from build123d import *

# Parameters (mm, degrees)
SKETCH1_W            = 25.4
SKETCH1_H            = 25.4
BOSS_EXTRUDE1_DEPTH  = 340.36
SKETCH2_W            = 22.225
SKETCH2_H            = 22.225
CUT_EXTRUDE1_DEPTH   = 681.72
SKETCH3_R            = 2.38125
CUT_EXTRUDE2_DEPTH   = 26.4
M6_CLEARANCE_HOLE1_D = 6.6


with BuildPart() as part:
    # Sketch1 → Boss-Extrude1 (new body, symmetric)
    with BuildSketch(Plane.XY):
        Rectangle(SKETCH1_W, SKETCH1_H)
    extrude(amount=BOSS_EXTRUDE1_DEPTH, both=True)

    # Sketch2 → Cut-Extrude1 (cut, through all)
    with BuildSketch(Plane.XY.offset(340.36)):
        Rectangle(SKETCH2_W, SKETCH2_H)
    extrude(amount=-CUT_EXTRUDE1_DEPTH, mode=Mode.SUBTRACT)

    # Sketch3 → Cut-Extrude2 (cut, through all)
    with BuildSketch(Plane(origin=(0, 12.7, 0), x_dir=(1, 0, 0), z_dir=(0, 1, 0))):
        with Locations((0, -215.9)):
            Circle(SKETCH3_R)
        with Locations((0, -203.2)):
            Circle(SKETCH3_R)
        with Locations((0, -190.5)):
            Circle(SKETCH3_R)
        with Locations((0, -177.8)):
            Circle(SKETCH3_R)
        with Locations((0, -165.1)):
            Circle(SKETCH3_R)
        with Locations((0, -152.4)):
            Circle(SKETCH3_R)
        with Locations((0, -139.7)):
            Circle(SKETCH3_R)
        with Locations((0, 139.7)):
            Circle(SKETCH3_R)
        with Locations((0, 152.4)):
            Circle(SKETCH3_R)
        with Locations((0, 165.1)):
            Circle(SKETCH3_R)
        with Locations((0, 177.8)):
            Circle(SKETCH3_R)
        with Locations((0, 190.5)):
            Circle(SKETCH3_R)
        with Locations((0, 215.9)):
            Circle(SKETCH3_R)
        with Locations((0, 203.2)):
            Circle(SKETCH3_R)
    extrude(amount=-CUT_EXTRUDE2_DEPTH, mode=Mode.SUBTRACT)

    # M6 Clearance Hole1 (through all)
    with Locations(Plane(origin=(0, 12.7, 0), x_dir=(1, 0, 0), z_dir=(0, 1, 0))):
        with Locations((0, 328.36), (0, -328.36)):
            Hole(M6_CLEARANCE_HOLE1_D / 2)


solid = part.part
For this review, take the finished solid that the model builds, in its own axes (mm). A direction names the side the tool comes from. Round coordinates to 2 decimals unless told otherwise and drop trailing zeros. Loops run counter-clockwise (first coordinate to the right, second up) from the corner with the lowest first, then second, coordinate; pieces in that order, holes last. Notation, with made-up numbers: (27, 48.5) - (56, 48.5) arc R17 cw to (56, 57.5) - close; hole circle Ø1 at (-31.5, -25). An arc over 180 degrees is marked (long way). One line per item, written item: value. Start each with the question number.
Item 1: Clearance check with a flat-ended pin moving along its axis: pin 1 Ø4 at (x, z) = (0, -328.36) entering from +Y. State where the tip first meets the part, or that it passes through.
Item 2: Take a section at A-A (y = -4.75). Give the boundary of the cut face in (x, z).
Item 3: Take a section at B-B (z = 288). Give the boundary of the cut face in (x, y), plus the area to 3 significant figures.
Item 4: For L1, parallel to X at y = 10.5, z = -31; L2, parallel to X at y = -11.85, z = 215.9, list the stretches that pass through material, from the lowest coordinate up.
Item 5: For faces 1 (the flat face through (12.7, 0, 5)), 2 (the flat face through (0, 11.112, 5)), list the 3-axis set-ups (+Z, -Z, +X, -X, +Y, -Y) from which the entire face can be reached by the end or side of a thin tool; tool diameter is ignored.
Item 6: The part is to be moulded in two halves that separate along Y. For faces 3 (the flat face through (-11.3, 0.1, 340.36)), 4 (the flat face through (-11.112, 0, 5)), 5 (the flat face through (0, 12.7, 5)), say which applies: +Y half, -Y half, draft (parallel to the pull), parting line (faces both ways), or undercut.
Answer below:
1. pin 1: passes through
2. outline: (-12.7, -340.36) - (-11.11, -340.36) - (-11.11, 340.36) - (-12.7, 340.36) - close; (11.11, -340.36) - (12.7, -340.36) - (12.7, 340.36) - (11.11, 340.36) - close
3. outline: (-12.7, -12.7) - (12.7, -12.7) - (12.7, 12.7) - (-12.7, 12.7) - close; hole (-11.11, -11.11) - (11.11, -11.11) - (11.11, 11.11) - (-11.11, 11.11) - close
3. area: 151 mm2
4. L1: x = -12.7 to -11.11, 11.11 to 12.7
4. L2: x = -12.7 to -2.38, 2.38 to 12.7
5. face 1: +Z, -Z, +X, +Y, -Y
5. face 2: +Z, -Z
6. face 3: draft
6. face 4: undercut
6. face 5: +Y half
